The listing builds one solid part. Answer for the finished solid, in the listing's coordinates (mm). Round coordinates to 2 decimals unless told otherwise and drop trailing zeros. Loops run counter-clockwise (first coordinate to the right, second up) from the corner with the lowest first, then second, coordinate; pieces in that order, holes last. Notation, with made-up numbers: M -6,69 L 39,69 A24 ccw 39,84 Z; hole C 67.25,82.5 d4. An arc over 180 degrees is marked long. Answer as a JSON object with one key per item and string values.
```python
from build123d import *
from build123d.topology import SkipClean

# Parameters (mm, degrees)
SKETCH1_W               = 15.24
SKETCH1_H               = 279.4
BOSS_EXTRUDE3_DEPTH     = 6.35
SKETCH2_R               = 2.75
CUT_EXTRUDE1_DEPTH      = 174.437553604
SKETCH3_W               = 15.24
SKETCH3_H               = 279.4
BOSS_EXTRUDE4_DEPTH     = 6.35
CUT_EXTRUDE2_DEPTH      = 174.437553604
CUT_EXTRUDE2_DEPTH_BACK = 174.437553604
SKETCH4_R               = 2.75


with BuildPart() as part:
    # Sketch1 → Boss-Extrude3 (new body)
    with BuildSketch(Plane.XY.offset(8)):
        with BuildLine():
            Line((-69.85, -152.4), (-44.45, -152.4))
            ThreePointArc((-44.45, -152.4), (-35.469743879, -148.680256121), (-31.75, -139.7))
            Line((-31.75, -139.7), (-31.75, 139.7))
            ThreePointArc((-31.75, 139.7), (-35.469743879, 148.680256121), (-44.45, 152.4))
            Line((-44.45, 152.4), (-69.85, 152.4))
            ThreePointArc((-69.85, 152.4), (-78.830256121, 148.680256121), (-82.55, 139.7))
            Line((-82.55, 139.7), (-82.55, -139.7))
            ThreePointArc((-82.55, -139.7), (-78.830256121, -148.680256121), (-69.85, -152.4))
        make_face()
        with Locations((-57.15, 0)):
            Rectangle(SKETCH1_W, SKETCH1_H, mode=Mode.SUBTRACT)
        with BuildLine():
            ThreePointArc((-44.45, -136.95), (-39.755456352, -135.005456352), (-41.7, -139.7))
            ThreePointArc((-41.7, -139.7), (-42.505456352, -137.755456352), (-44.45, -136.95))
        make_face(mode=Mode.SUBTRACT)
        with BuildLine():
            ThreePointArc((-72.6, -139.7), (-74.544543648, -135.005456352), (-69.85, -136.95))
            ThreePointArc((-69.85, -136.95), (-71.794543648, -137.755456352), (-72.6, -139.7))
        make_face(mode=Mode.SUBTRACT)
        with BuildLine():
            ThreePointArc((-41.7, 139.7), (-39.755456352, 135.005456352), (-44.45, 136.95))
            ThreePointArc((-44.45, 136.95), (-42.505456352, 137.755456352), (-41.7, 139.7))
        make_face(mode=Mode.SUBTRACT)
        with BuildLine():
            ThreePointArc((-69.85, 136.95), (-74.544543648, 135.005456352), (-72.6, 139.7))
            ThreePointArc((-72.6, 139.7), (-71.794543648, 137.755456352), (-69.85, 136.95))
        make_face(mode=Mode.SUBTRACT)
    extrude(amount=-BOSS_EXTRUDE3_DEPTH)

    # Sketch2 → Cut-Extrude1 (cut, through all)
    with SkipClean():  # the faces are left unmerged after this step: merging them gives an invalid solid
        with BuildSketch(Plane.XY.offset(8)):
            with Locations(Location((-41.7, 136.95, 0), (0, 0, 180))):
                Circle(SKETCH2_R)
            with Locations(Location((-72.6, 136.95, 0), (0, 0, 180))):
                Circle(SKETCH2_R)
            with Locations(Location((-41.7, -136.95, 0), (0, 0, 180))):
                Circle(SKETCH2_R)
            with Locations(Location((-72.6, -136.95, 0), (0, 0, 180))):
                Circle(SKETCH2_R)
        extrude(amount=-CUT_EXTRUDE1_DEPTH, mode=Mode.SUBTRACT)

    # Sketch3 → Boss-Extrude4 (add)
    with SkipClean():  # the faces are left unmerged after this step: merging them gives an invalid solid
        with BuildSketch(Plane.XY.offset(8)):
            with Locations((-57.15, 0)):
                Rectangle(SKETCH3_W, SKETCH3_H)
        extrude(amount=-BOSS_EXTRUDE4_DEPTH)

    # Sketch4 → Cut-Extrude2 (cut, two sides: drawn at the far end of the back side and taken through both)
    with SkipClean():  # the faces are left unmerged after this step: merging them gives an invalid solid
        with BuildSketch(Plane(origin=(0, 0, 1.65), x_dir=(-1, 0, 0), z_dir=(0, 0, -1)).offset(-CUT_EXTRUDE2_DEPTH_BACK)):
            with Locations((47.2, 16.3)):
                Circle(SKETCH4_R)
            with Locations((67.1, 16.3)):
                Circle(SKETCH4_R)
            with Locations((47.2, -16.3)):
                Circle(SKETCH4_R)
            with Locations((67.1, -16.3)):
                Circle(SKETCH4_R)
        extrude(amount=CUT_EXTRUDE2_DEPTH + CUT_EXTRUDE2_DEPTH_BACK, mode=Mode.SUBTRACT)


solid = part.part
```
Item 1: The part is cut by section B-B (y = -16.3). Give the vertices of the cut face in (x, z), then the cut area to 3 significant figures.
Values follow:
{"outline": "M -82.55,1.65 L -69.85,1.65 L -69.85,8 L -82.55,8 Z; M -64.35,1.65 L -49.95,1.65 L -49.95,8 L -64.35,8 Z; M -44.45,1.65 L -31.75,1.65 L -31.75,8 L -44.45,8 Z", "area": "253 mm^2"}
Item 2: The part is cut by section D-D (x = -78). Give the vertices of the cut face in (y, z), then the cut area to 3 significant figures.
Values follow:
{"outline": "M -149.44,1.65 L 149.44,1.65 L 149.44,8 L -149.44,8 Z", "area": "1,900 mm^2"}
Item 3: A flat-ended cylindrical pin translates along its axis: P1, Ø5, axis at x = -72.6, y = 136.95, coming from the -Z side. Find the tip coordinate at first contact, or state that the pin passes through.
Values follow:
{"P1": "through"}
Item 4: Straight lines are drawn through the part: line 1 (Y direction, x = -47.2, z = 3.5); line 2 (X direction, y = 136.95, z = 4.75); line 3 (X direction, y = 18, z = 3.5). For each, find the intervals that lie inside material, in ascending order.
Values follow:
{"line 1": "-152.4 to -19.05, -13.55 to 13.55, 19.05 to 152.4", "line 2": "-82.55 to -75.35, -69.85 to -44.45, -38.95 to -31.75", "line 3": "-82.55 to -69.26, -64.94 to -49.36, -45.04 to -31.75"}
Item 5: The part is cut by section C-C (z = 6.75). Give the number of separate pieces and of enclosed holes in the cut face, then the cut area to 3 significant figures.
Values follow:
{"separate pieces": "1", "enclosed holes": "8", "area": "15,200 mm^2"}
Item 6: The part is cut by section A-A (x = -67.1). Give the vertices of the cut face in (y, z).
Values follow:
{"outline": "M -152.4,1.65 L -19.05,1.65 L -19.05,8 L -152.4,8 Z; M -13.55,1.65 L 13.55,1.65 L 13.55,8 L -13.55,8 Z; M 19.05,1.65 L 152.4,1.65 L 152.4,8 L 19.05,8 Z"}
Item 7: Determine the mould class of faces 1 (the face through (-69.64, 15.25, 4.87)), 2 (the face through (-58, 2, 1.65)), 3 (the face through (-57, -152.4, 5)) for opening direction Y: released by +Y, released by -Y, zero draft, split by the parting line, or undercut.
Values follow:
{"face 1": "undercut", "face 2": "zero draft", "face 3": "released by -Y"}
